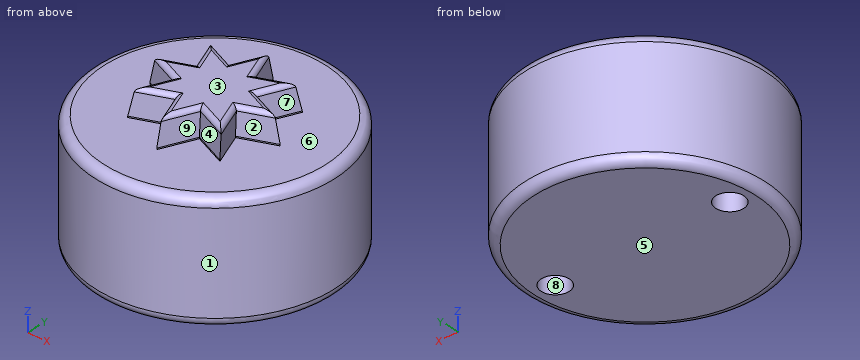
```python
from build123d import *

# Parameters (mm, degrees)
F0_R     = 26.5
F0_R_2   = 3.1
F1_DEPTH = 20
F2_R     = 26.5
F3_DEPTH = 6
F4_R     = 2
F6_DEPTH = 6
F7_SIZE2 = 5.7150261514
F7_SIZE  = 0.5
F8_SIZE2 = 5.7150261514
F8_SIZE  = 0.5
F9_R     = 1


with BuildPart() as f1:
    # F0 (on Top) → F1 (new body)
    with BuildSketch(Plane.XY):
        Circle(F0_R)
        with Locations((-19.7989898732, 0.6299423149)):
            Circle(F0_R_2, mode=Mode.SUBTRACT)
        with Locations((19.7989898732, 0.6299423149)):
            Circle(F0_R_2, mode=Mode.SUBTRACT)
    extrude(amount=F1_DEPTH)

    # F2 (on face) → F3 (join)
    with BuildSketch(Plane.XY.offset(20)):
        Circle(F2_R)
    extrude(amount=F3_DEPTH)

    # F4
    f4_edges = [f1.edges().sort_by_distance(p)[0] for p in [
        (-26.5, 0, 26),
        (-26.5, 0, 0),
    ]]
    fillet(f4_edges, radius=F4_R)

    # F5 (on face) → F6 (join)
    with BuildSketch(Plane.XY.offset(26)):
        Polygon((0, 14.7820725202), (-3.0614674589, 7.3910362601), (-10.452503719, 10.452503719), (-7.3910362601, 3.0614674589), (-14.7820725202, 0), (-7.3910362601, -3.0614674589), (-10.452503719, -10.452503719), (-3.0614674589, -7.3910362601), (0, -14.7820725202), (3.0614674589, -7.3910362601), (10.452503719, -10.452503719), (7.3910362601, -3.0614674589), (14.7820725202, 0), (7.3910362601, 3.0614674589), (10.452503719, 10.452503719), (3.0614674589, 7.3910362601), align=None)
    extrude(amount=F6_DEPTH)

    # F7
    f7_edges = [f1.edges().sort_by_distance(p)[0] for p in [
        (6.756986, -8.92177, 32),
        (-1.530734, -11.086554, 32),
        (-8.92177, -6.756986, 32),
        (-11.086554, 1.530734, 32),
        (-6.756986, 8.92177, 32),
        (1.530734, 11.086554, 32),
        (8.92177, 6.756986, 32),
        (11.086554, -1.530734, 32),
    ]]
    f7_side = f1.faces().sort_by_distance((0, 0, 32))[0]
    chamfer(f7_edges, length=F7_SIZE, length2=F7_SIZE2, reference=f7_side)

    # F8
    f8_edges = [f1.edges().sort_by_distance(p)[0] for p in [
        (1.666033, -10.759914, 32),
        (-6.430345, -8.786471, 32),
        (-10.759914, -1.666033, 32),
        (-8.786471, 6.430345, 32),
        (-1.666033, 10.759914, 32),
        (6.430345, 8.786471, 32),
        (10.759914, 1.666033, 32),
    ]]
    f8_side = f1.faces().sort_by_distance((0, 0, 32))[0]
    chamfer(f8_edges, length=F8_SIZE, length2=F8_SIZE2, reference=f8_side)

    # F9
    f9_edges = [f1.edges().sort_by_distance(p)[0] for p in [
        (10.337602, -1.299764, 32),
        (10.337602, 1.299764, 32),
        (7.295365, -2.830498, 32),
        (6.968725, 2.695199, 32),
        (8.786471, -6.430345, 32),
        (6.833426, 3.021839, 32),
        (6.717357, -8.364159, 32),
        (8.22886, 6.390717, 32),
        (3.021839, -6.833426, 32),
        (6.390717, 8.22886, 32),
        (2.695199, -6.968725, 32),
        (3.021839, 6.833426, 32),
        (1.299764, -10.337602, 32),
        (2.695199, 6.968725, 32),
        (-1.299764, -10.337602, 32),
        (1.299764, 10.337602, 32),
        (-2.695199, -6.968725, 32),
        (-1.299764, 10.337602, 32),
        (-3.021839, -6.833426, 32),
        (-2.695199, 6.968725, 32),
        (-6.390717, -8.22886, 32),
        (-3.021839, 6.833426, 32),
        (-8.22886, -6.390717, 32),
        (-6.390717, 8.22886, 32),
        (-6.833426, -3.021839, 32),
        (-8.22886, 6.390717, 32),
        (-6.968725, -2.695199, 32),
        (-6.833426, 3.021839, 32),
        (-10.337602, -1.299764, 32),
        (-6.968725, 2.695199, 32),
        (-10.337602, 1.299764, 32),
    ]]
    fillet(f9_edges, radius=F9_R)


solid = f1.part
```
CAD build for the part. Positions are in the model's coordinates, mm. Face numbers are marked on the shaded views. A direction names the side the tool comes from. Round coordinates to 2 decimals unless told otherwise and drop trailing zeros. Order: outer loops, then holes, each group sorted by start corner. A loop starts at its lowest first (then second) coordinate and runs counter-clockwise, first axis right, second up.
Q1. Which spindle directions (+Z, -Z, +X, -X, +Y, -Y) get a long thin tool onto all of the face, cutting with end or side? Do the marked faces 5, 6, 7, 8 and 9. Say none if no direction does.
Q2. Two-plate mould, pull along Y, no slides. Class the marked faces 1, 2, 3 and 4: pulls with the +Y half, pulls with the -Y half, needs draft (parallel to the pull), parting line crosses it, or undercut.
Q3. Wall check: L1, parallel to X at y = -1.5, z = 10.5; L2, parallel to Y at x = -7.5, z = 28; L3, parallel to Z at x = -17, y = -9. Give the ranges that are in metal, low to high.
Q4. Drop flat-ended pins along their axis: pin 1 (10 mm diameter, centred on x = -19.8, y = 0.63, fed in from -Z); pin 2 (3 mm diameter, centred on y = 2.5, z = 14, fed in from -X); pin 3 (2 mm diameter, centred on x = 12.5, z = 4.5, fed in from -Y); pin 4 (10 mm diameter, centred on x = -5.5, z = 12.5, fed in from +Y). Give the stop position or say it passes through.
Q5. Slice it at A-A (z = 27). Write the cut outline in (x, y).
Q6. Slice it at B-B (z = 8). Write the cut outline in (x, y).
Results below:
1. face 5: -Z, +X, -X, +Y, -Y
1. face 6: +Z
1. face 7: +Z, +X
1. face 8: -Z
1. face 9: +Z, -Y
2. face 1: parting line crosses it
2. face 2: undercut
2. face 3: needs draft
2. face 4: pulls with the -Y half
3. L1: x = -26.46 to -22.05, -17.55 to 17.55, 22.05 to 26.46
3. L2: y = -9.07 to -3.72, -2.85 to 2.85, 3.72 to 9.07
3. L3: z = 0 to 26
4. pin 1: stops at z = 0
4. pin 2: stops at x = -26.48
4. pin 3: stops at y = -23.87
4. pin 4: stops at y = 26.5
5. outline: (-14.62, 0) - (-7.31, -3.03) - (-10.34, -10.34) - (-3.03, -7.31) - (0, -14.62) - (3.03, -7.31) - (10.42, -10.37) - (7.37, -3) - (14.62, 0) - (7.31, 3.03) - (10.34, 10.34) - (3.03, 7.31) - (0, 14.62) - (-3.03, 7.31) - (-10.34, 10.34) - (-7.31, 3.03) - close
6. outline: circle Ø53 at (0, 0); hole circle Ø6.2 at (-19.8, 0.63); hole circle Ø6.2 at (19.8, 0.63)
